The model under review builds one solid part; all positions refer to its coordinate system, in mm. A direction names the side the tool comes from. Coordinates: 2 decimals unless noted, no trailing zeros. Write each loop counter-clockwise with the first axis right and the second up, starting at its lowest first coordinate (ties: lowest second). Pieces come first, ordered by that corner, then holes.
1) Mouldability with a two-part tool opening along Y and no side actions: class faces 4 (the flat face through (49.1, 10, -3)), 5 (the cylindrical face through (64.6, 0.86, -3.45)), 6 (the flat face through (0, 10, -13)) as released by +Y, released by -Y, zero draft, split by the parting line, or undercut.
2) Add section C-C, the plane y = 10.75. Give the number of separate pieces and of enclosed holes in the cut face, then the cut area to 3 significant figures.
3) For P1, Ø8.5, axis at x = 35, y = 10, coming from the +Z side; P2, Ø6, axis at x = 53, y = 12.5, coming from the -Z side, all flat-tipped, find the tip position at first contact; note any pin that passes through.
4) Add section A-A, the plane x = 8. State the section outline as (y, z) points.
5) Machinability: for faces 1 (the flat face through (61.9, 10, -3)), 2 (the flat face through (42.5, 10, -16)), 3 (the cylindrical face through (3.24, 6.35, -6.9)), which of the approach directions +Z, -Z, +X, -X, +Y, -Y give a long, thin tool a straight path to every point of the face, cutting with its end or side? Answer none if there is none.
6) For line 1 (Y direction, x = 35, z = -20); line 2 (Y direction, x = 8, z = -7.25); line 3 (X direction, y = 14, z = -22.5), list the stretches that pass through material, from the lowest coordinate up.
7) Add section B-B, the plane z = -3.5. State the section outline as (x, y) points.
8) Add section D-D, the plane z = -16.5. State the section outline as (x, y) points.
from build123d import *

# Parameters (mm, degrees)
SKETCH1_R           = 2.6
BOSS_EXTRUDE1_DEPTH = 7
BOSS_EXTRUDE2_DEPTH = 19
SKETCH3_R           = 2.6
CUT_EXTRUDE1_DEPTH  = 19
SKETCH4_R           = 6
CUT_EXTRUDE2_DEPTH  = 14


with BuildPart() as part:
    # Sketch1 → Boss-Extrude1 (new body)
    with BuildSketch(Plane.XY):
        with BuildLine():
            Line((3, 0), (62.5, 0))
            ThreePointArc((62.5, 0), (64.621320344, 0.878679656), (65.5, 3))
            Line((65.5, 3), (65.5, 17))
            ThreePointArc((65.5, 17), (64.621320344, 19.121320344), (62.5, 20))
            Line((62.5, 20), (3, 20))
            ThreePointArc((3, 20), (0.878679656, 19.121320344), (0, 17))
            Line((0, 17), (0, 3))
            ThreePointArc((0, 3), (0.878679656, 0.878679656), (3, 0))
        make_face()
        with Locations((8, 10)):
            Circle(SKETCH1_R, mode=Mode.SUBTRACT)
        with Locations((35, 10)):
            Circle(SKETCH1_R, mode=Mode.SUBTRACT)
        with BuildLine():
            Line((49.1, 15.4), (49.1, 4.6))
            ThreePointArc((49.1, 4.6), (50.7, 3), (52.3, 4.6))
            Line((52.3, 4.6), (52.3, 15.4))
            ThreePointArc((52.3, 15.4), (50.7, 17), (49.1, 15.4))
        make_face(mode=Mode.SUBTRACT)
        with BuildLine():
            Line((58.7, 15.4), (58.7, 4.6))
            ThreePointArc((58.7, 4.6), (60.3, 3), (61.9, 4.6))
            Line((61.9, 4.6), (61.9, 15.4))
            ThreePointArc((61.9, 15.4), (60.3, 17), (58.7, 15.4))
        make_face(mode=Mode.SUBTRACT)
    extrude(amount=-BOSS_EXTRUDE1_DEPTH)

    # Sketch2 → Boss-Extrude2 (add)
    with BuildSketch(Plane(origin=(0, 0, -7), x_dir=(-1, 0, 0), z_dir=(0, 0, -1))):
        with BuildLine():
            Line((-42.5, 20), (-42.5, 0))
            Line((-42.5, 0), (-3, 0))
            ThreePointArc((-3, 0), (-0.878679656, 0.878679656), (0, 3))
            Line((0, 3), (0, 17))
            ThreePointArc((0, 17), (-0.878679656, 19.121320344), (-3, 20))
            Line((-3, 20), (-42.5, 20))
        make_face()
    extrude(amount=BOSS_EXTRUDE2_DEPTH)

    # Sketch3 → Cut-Extrude1 (cut)
    with BuildSketch(Plane.XY.offset(-7)):
        with Locations((8, 10)):
            Circle(SKETCH3_R)
        with Locations((35, 10)):
            Circle(SKETCH3_R)
    extrude(amount=-CUT_EXTRUDE1_DEPTH, mode=Mode.SUBTRACT)

    # Sketch4 → Cut-Extrude2 (cut)
    with BuildSketch(Plane.XY):
        with Locations((8, 10)):
            Circle(SKETCH4_R)
        with Locations((35, 10)):
            Circle(SKETCH4_R)
    extrude(amount=-CUT_EXTRUDE2_DEPTH, mode=Mode.SUBTRACT)


solid = part.part
Geometry results:
1. face 4: undercut
1. face 5: released by -Y
1. face 6: zero draft
2. separate pieces: 5
2. enclosed holes: 0
2. area: 768 mm2
3. P1: stops at z = -14
3. P2: stops at z = -7
4. outline: (0, -26) - (7.4, -26) - (7.4, -14) - (4, -14) - (4, 0) - (0, 0) - close; (12.6, -26) - (20, -26) - (20, 0) - (16, 0) - (16, -14) - (12.6, -14) - close
5. face 1: +Z, -Z
5. face 2: -Z, +X, +Y, -Y
5. face 3: +Z
6. line 1: y = 0 to 7.4, 12.6 to 20
6. line 2: y = 0 to 4, 16 to 20
6. line 3: x = 0 to 42.5
7. outline: (0, 3) arc R3 ccw to (3, 0) - (62.5, 0) arc R3 ccw to (65.5, 3) - (65.5, 17) arc R3 ccw to (62.5, 20) - (3, 20) arc R3 ccw to (0, 17) - close; hole circle Ø12 at (8, 10); hole circle Ø12 at (35, 10); hole (49.1, 4.6) arc R1.6 ccw to (52.3, 4.6) - (52.3, 15.4) arc R1.6 ccw to (49.1, 15.4) - close; hole (58.7, 4.6) arc R1.6 ccw to (61.9, 4.6) - (61.9, 15.4) arc R1.6 ccw to (58.7, 15.4) - close
8. outline: (0, 3) arc R3 ccw to (3, 0) - (42.5, 0) - (42.5, 20) - (3, 20) arc R3 ccw to (0, 17) - close; hole circle Ø5.2 at (8, 10); hole circle Ø5.2 at (35, 10)
